For this review, take the finished solid that the model builds, in its own axes (mm). A direction names the side the tool comes from. Give positions to 0.01 mm unless a question says otherwise; leave off trailing zeros. Write each loop counter-clockwise with the first axis right and the second up, starting at its lowest first coordinate (ties: lowest second). Pieces come first, ordered by that corner, then holes. Notation, with made-up numbers: M 62,66 L 90,66 A20 cw 90,91 Z; hole C 68.5,39.25 d11. An arc over 180 degrees is marked long. Write item = value, one per line.
```python
from build123d import *

# Parameters (mm, degrees)
F0_R      = 20
F1_DEPTH  = 15
F2_R      = 18
F3_DEPTH  = 13
F4_R      = 3.5
F4_R_2    = 1.5
F5_DEPTH  = 13
F6_R      = 3.5
F6_R_2    = 1.5
F7_DEPTH  = 3
F10_DEPTH = 2


with BuildPart() as f1:
    # F0 (on Top) → F1 (new body)
    with BuildSketch(Plane.XY):
        Circle(F0_R)
    extrude(amount=F1_DEPTH)

    # F2 (on face) → F3 (cut)
    with BuildSketch(Plane.XY.offset(15)):
        Circle(F2_R)
    extrude(amount=-F3_DEPTH, mode=Mode.SUBTRACT)

    # F4 (on face) → F5 (join)
    with BuildSketch(Plane.XY.offset(15)):
        Circle(F4_R)
        Circle(F4_R_2, mode=Mode.SUBTRACT)
    extrude(amount=-F5_DEPTH)

    # F6 (on face) → F7 (join)
    with BuildSketch(Plane.XY.offset(15)):
        Circle(F6_R)
        Circle(F6_R_2, mode=Mode.SUBTRACT)
    extrude(amount=F7_DEPTH)

    # F9 (on face) → F10 (cut)
    with BuildSketch(Plane(origin=(0, 0, 0), x_dir=(1, 0, 0), z_dir=(0, 0, -1))):
        with BuildLine():
            Line((-2.9190978863, 4.0177935548), (-1.6146279111, 17.9274364232))
            ThreePointArc((-1.6146279111, 17.9274364232), (-10.5801345413, 14.5623058987), (-16.5510577667, 7.0754849166))
            Line((-16.5510577667, 7.0754849166), (-2.9190978863, 4.0177935548))
        make_face()
        with BuildLine():
            ThreePointArc((-17.5489526949, 4.0042801241), (-17.1190172933, -5.5623058987), (-11.8437441606, -13.5545462579))
            Line((-11.8437441606, -13.5545462579), (-4.7231995965, -1.5346605781))
            Line((-4.7231995965, -1.5346605781), (-17.5489526949, 4.0042801241))
        make_face()
        with BuildLine():
            ThreePointArc((-9.2312213213, -15.452655206), (0, -18), (9.2312213213, -15.452655206))
            Line((9.2312213213, -15.452655206), (0, -4.9662659533))
            Line((0, -4.9662659533), (-9.2312213213, -15.452655206))
        make_face()
        with BuildLine():
            ThreePointArc((11.8437441606, -13.5545462579), (16.3888284342, -7.4435409957), (18, 0))
            ThreePointArc((18, 0), (17.8868827428, 2.0148016642), (17.5489526949, 4.0042801241))
            Line((17.5489526949, 4.0042801241), (4.7231995965, -1.5346605781))
            Line((4.7231995965, -1.5346605781), (11.8437441606, -13.5545462579))
        make_face()
        with BuildLine():
            Line((2.9190978863, 4.0177935548), (16.5510577667, 7.0754849166))
            ThreePointArc((16.5510577667, 7.0754849166), (10.5801345413, 14.5623058987), (1.6146279111, 17.9274364232))
            Line((1.6146279111, 17.9274364232), (2.9190978863, 4.0177935548))
        make_face()
        with BuildLine():
            Line((-1.3322676027, -3.4528501024), (-1.6587573928, -3.0819675391))
            ThreePointArc((-1.6587573928, -3.0819675391), (-2.057248383, -2.8315594803), (-2.4185410871, -2.5299523731))
            Line((-2.4185410871, -2.5299523731), (-2.8721622593, -2.3340511457))
            Line((-2.8721622593, -2.3340511457), (-8.0671256706, -11.1034459232))
            Line((-8.0671256706, -11.1034459232), (-1.3322676027, -3.4528501024))
        make_face()
        with BuildLine():
            Line((2.8721622593, -2.3340511457), (2.4185410871, -2.5299523731))
            ThreePointArc((2.4185410871, -2.5299523731), (2.057248383, -2.8315594803), (1.6587573928, -3.0819675391))
            Line((1.6587573928, -3.0819675391), (1.3322676027, -3.4528501024))
            Line((1.3322676027, -3.4528501024), (8.0671256706, -11.1034459232))
            Line((8.0671256706, -11.1034459232), (2.8721622593, -2.3340511457))
        make_face()
        with BuildLine():
            ThreePointArc((3.1534979878, 1.5183709826), (3.328697807, 1.0815594803), (3.443709535, 0.6251916817))
            Line((3.443709535, 0.6251916817), (3.6955489199, 0.2000724244))
            Line((3.6955489199, 0.2000724244), (13.0528835265, 4.2411389504))
            Line((13.0528835265, 4.2411389504), (3.1073615002, 2.0103271628))
            Line((3.1073615002, 2.0103271628), (3.1534979878, 1.5183709826))
        make_face()
        with BuildLine():
            ThreePointArc((-0.4695721472, 3.4683572478), (0, 3.5), (0.4695721472, 3.4683572478))
            Line((0.4695721472, 3.4683572478), (0.9517072369, 3.5765016608))
            Line((0.9517072369, 3.5765016608), (0, 13.7246139455))
            Line((0, 13.7246139455), (-0.9517072369, 3.5765016608))
            Line((-0.9517072369, 3.5765016608), (-0.4695721472, 3.4683572478))
        make_face()
        with BuildLine():
            ThreePointArc((-3.443709535, 0.6251916817), (-3.328697807, 1.0815594803), (-3.1534979878, 1.5183709826))
            Line((-3.1534979878, 1.5183709826), (-3.1073615002, 2.0103271628))
            Line((-3.1073615002, 2.0103271628), (-13.0528835265, 4.2411389504))
            Line((-13.0528835265, 4.2411389504), (-3.6955489199, 0.2000724244))
            Line((-3.6955489199, 0.2000724244), (-3.443709535, 0.6251916817))
        make_face()
    extrude(amount=-F10_DEPTH, mode=Mode.SUBTRACT)


solid = f1.part
```
1. We need section D-D, the plane y = -12.5. Write out the cut boundary in (x, z), then the cut area to 3 significant figures.
Responses:
outline = M -15.61,0 L -12.95,0 L -12.95,15 L -15.61,15 Z; M -2.12,0 L -0.11,0 L -0.11,2 L -2.12,2 Z; M 0.11,0 L 2.12,0 L 2.12,2 L 0.11,2 Z; M 12.95,0 L 15.61,0 L 15.61,15 L 12.95,15 Z
area = 87.9 mm2
2. The part is to be moulded in two halves that separate along Y. For faces 3 (the face through (0, 0, 2)), 4 (the face through (0, -2, 18)), say which applies: +Y half, -Y half, draft (parallel to the pull), parting line (faces both ways), or undercut.
Responses:
face_3 = undercut
face_4 = draft
3. Machinability: for faces 1 (the face through (-1.5, 0.07, 9.89)), 2 (the face through (-8.333, 7.629, 0.986)), which of the approach directions +Z, -Z, +X, -X, +Y, -Y give a long, thin tool a straight path to every point of the face, cutting with its end or side? Answer none if there is none.
Responses:
face_1 = +Z
face_2 = +Z, -Z
4. Insertion check: P1, Ø10, axis at x = -10.5, y = 0, coming from the +Z side; P2, Ø4, axis at x = 15, y = 14.5, coming from the +Z side; P3, Ø1.5, axis at x = -8, z = 14.5, coming from the -Y side. Each pin has a flat end and moves straight along its axis. Give the tip position at first contact, or say it passes through.
Responses:
P1 = 2
P2 = 15
P3 = -18.64
5. We need section B-B, the plane z = 10. Write out the cut boundary in (x, y).
Responses:
outline = C 0,0 d40; C 0,0 d7; hole C 0,0 d36; hole C 0,0 d3
6. We need section A-A, the plane y = 1. Write out the cut boundary in (x, z).
Responses:
outline = M -19.97,0 L -17.97,0 L -17.97,15 L -19.97,15 Z; M -5.96,0 L 5.96,0 L 5.96,2 L 3.35,2 L 3.35,18 L 1.12,18 L 1.12,2 L -1.12,2 L -1.12,18 L -3.35,18 L -3.35,2 L -5.96,2 Z; M 17.97,0 L 19.97,0 L 19.97,15 L 17.97,15 Z
7. We need section C-C, the plane x = -7. Write out the cut boundary in (y, z) (3 decimals), then the cut area to 3 significant figures.
Responses:
outline = M -18.735,0 L -16.583,0 L -16.583,15 L -18.735,15 Z; M -4.933,0 L -2.883,0 L -2.883,2 L -4.933,2 Z; M -1.627,0 L 0.551,0 L 0.551,2 L -1.627,2 Z; M 5.378,0 L 9.302,0 L 9.302,2 L 5.378,2 Z; M 9.891,0 L 12.918,0 L 12.918,2 L 9.891,2 Z; M 16.583,0 L 18.735,0 L 18.735,15 L 16.583,15 Z
area = 86.9 mm2
8. For line 1 along Y through (x, z) = (0, 12.75); line 2 along X through (y, z) = (-10.5, 1.5); line 3 along Z through (x, y) = (3, -2.5), list the stretches that pass through material, from the lowest coordinate up. Write a range as from..to.
Responses:
line_1 = -20..-18, -3.5..-1.5, 1.5..3.5, 18..20
line_2 = -17.02..-14.62, -2.31..-0.3, 0.3..2.31, 14.62..17.02
line_3 = 0..2
